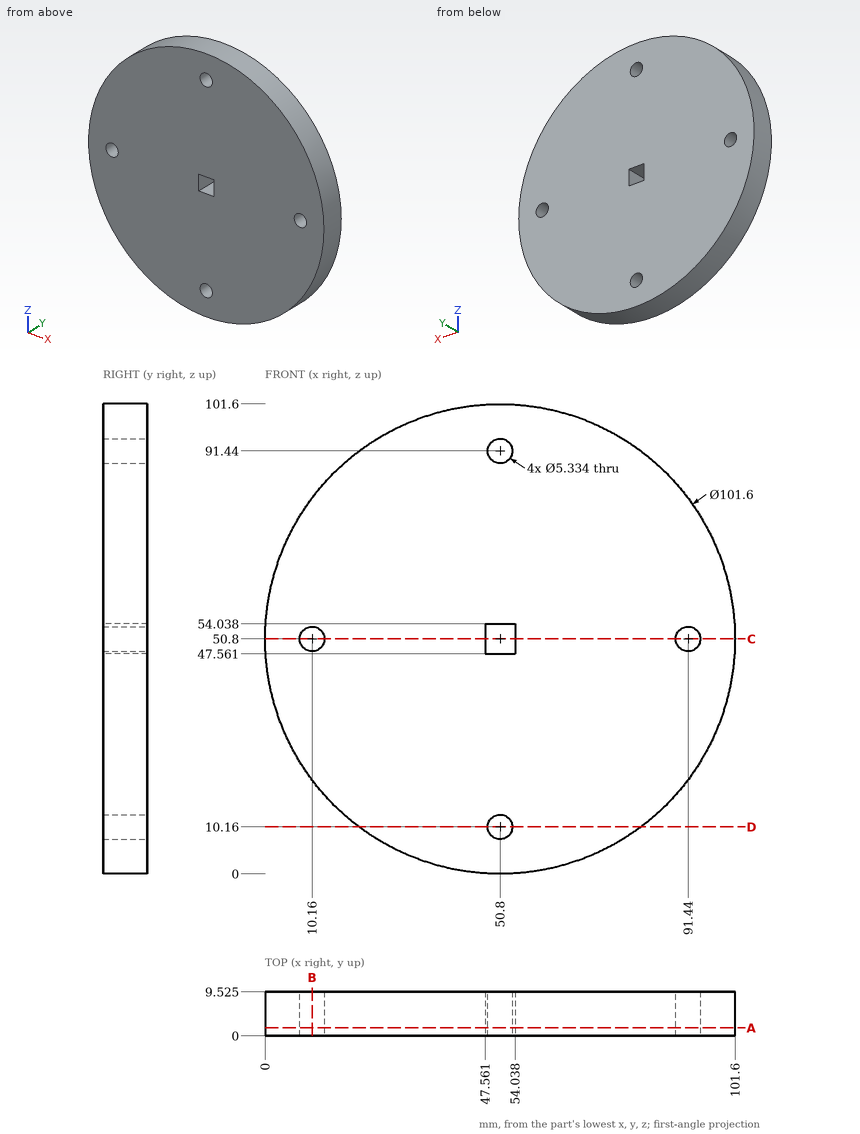
Geometry: see drawing. Coordinates: mm, zero at the bounding-box minimum. Give positions to 0.01 mm unless a question says otherwise; leave off trailing zeros. Order: outer loops, then holes, each group sorted by start corner. A loop starts at its lowest first (then second) coordinate and runs counter-clockwise, first axis right, second up. Notation, with made-up numbers: M 33,80 L 72,80 A7 cw 72,85 Z; hole C -11.75,32.25 d1. An arc over 180 degrees is marked long. Answer as CSV lines item,"result". Start each with the question number.
1) Cut plane C-C (z = 50.8). Output: boundary loops of the cut face in (x, y) (1 decimal).
2) Cut plane A-A (y = 1.75). Output: boundary loops of the cut face in (x, z) (1 decimal).
3) Cut plane B-B (x = 10.16). Output: boundary loops of the cut face in (y, z) (1 decimal), then the cut area to 3 significant figures.
4) First-contact query: P1, Ø3, axis at y = 8, z = 55, coming from the -X side; P2, Ø3, axis at x = 51.5, y = 5.5, coming from the -Z side; P3, Ø5, axis at x = 51.5, y = 2.5, coming from the +Z side. Flat tips, straight axial feed; report the tip coordinate or a pass-through.
5) Cut plane D-D (z = 10.16). Output: boundary loops of the cut face in (x, y) (1 decimal), then the cut area to 3 significant figures.
6) Line query: line 1 (X direction, y = 6.5, z = 50.8); line 2 (X direction, y = 3.5, z = 10.16) (1 decimal). Output: solid intervals per line, ascending. Write a range as from..to.
Findings below:
1,outline,"M 0,0 L 7.5,0 L 7.5,9.5 L 0,9.5 Z; M 12.8,0 L 47.6,0 L 47.6,9.5 L 12.8,9.5 Z; M 54,0 L 88.8,0 L 88.8,9.5 L 54,9.5 Z; M 94.1,0 L 101.6,0 L 101.6,9.5 L 94.1,9.5 Z"
2,outline,"C 50.8,50.8 d101.6; hole C 10.2,50.8 d5.3; hole M 47.6,47.6 L 54,47.6 L 54,54 L 47.6,54 Z; hole C 50.8,10.2 d5.3; hole C 50.8,91.4 d5.3; hole C 91.4,50.8 d5.3"
3,outline,"M 0,20.3 L 9.5,20.3 L 9.5,48.1 L 0,48.1 Z; M 0,53.5 L 9.5,53.5 L 9.5,81.3 L 0,81.3 Z"
3,area,"530 mm²"
4,P1,"stops at x = 0.07"
4,P2,"stops at z = 0"
4,P3,"stops at z = 101.6"
5,outline,"M 20.3,0 L 48.1,0 L 48.1,9.5 L 20.3,9.5 Z; M 53.5,0 L 81.3,0 L 81.3,9.5 L 53.5,9.5 Z"
5,area,"530 mm²"
6,line 1,"x = 0..7.49, 12.83..47.56, 54.04..88.77, 94.11..101.6"
6,line 2,"x = 20.3..48.1, 53.5..81.3"
